Verification items for the finished model (mm, model axes). Face numbers are marked on the shaded views. A direction names the side the tool comes from. Give positions to 0.01 mm unless a question says otherwise; leave off trailing zeros. Write each loop counter-clockwise with the first axis right and the second up, starting at its lowest first coordinate (ties: lowest second). Pieces come first, ordered by that corner, then holes. Notation, with made-up numbers: (57.5, 83.25) - (66.5, 83.25) arc R8 ccw to (66.5, 93.25) - close; hole circle Ø10 at (82.25, 86). An arc over 180 degrees is marked (long way). Answer as a JSON object with one key per item and string values. Group by question number.
Item 1: Go/stop test with flat-tipped pins: pin 1 (3 mm diameter, centred on x = -6.5, y = -8, fed in from +Z); pin 2 (1 mm diameter, centred on y = -6, z = 33.5, fed in from -X); pin 3 (12 mm diameter, centred on x = 6, y = 8.5, fed in from +Z). Record where each tip stops, or that it passes through.
Item 2: Sectioned sample at D-D, the plane z = 50. Record the boundary of the cut face in (x, y), and give its area (3 significant figures).
Item 3: Sectioned sample at A-A, the plane x = 0. Record the boundary of the cut face in (y, z).
Item 4: Tool access check on the marked faces 1 and 2. Record the directions out of +Z, -Z, +X, -X, +Y, -Y that give a thin tool (end or side, any length) a straight path to the whole face; none if there is none.
Item 5: Scan lines: line 1 along Z through (x, y) = (11.5, 4.75); line 2 along Z through (x, y) = (-0.5, 3.5); line 3 along Y through (x, z) = (-8, 40.8). Record each from-to range of solid material in increasing order. Write a range as [from, to].
Item 6: Sectioned sample at B-B, the plane z = 14.5. Record the boundary of the cut face in (x, y), and give its area (3 significant figures).
Item 7: Sectioned sample at C-C, the plane y = 12.25. Record the boundary of the cut face in (x, z), and give its area (3 significant figures).
```python
from build123d import *

# Parameters (mm, degrees)
F0_R     = 14
F1_DEPTH = 42
F2_R     = 5
F3_DEPTH = 2.2
F4_R     = 2.25
F5_DEPTH = 17.25
F6_D     = 2.2
F6_DEPTH = 4
F6_TIP   = 0.6609466809


with BuildPart() as f1:
    # F0 (on Top) → F1 (new body)
    with BuildSketch(Plane.XY):
        Circle(F0_R)
    extrude(amount=F1_DEPTH)

    # F2 (on face) → F3 (join)
    with BuildSketch(Plane.XY.offset(42)):
        Circle(F2_R)
    extrude(amount=F3_DEPTH)

    # F4 (on face) → F5 (join)
    with BuildSketch(Plane.XY.offset(44.2)):
        Circle(F4_R)
    extrude(amount=F5_DEPTH)

    # F6
    with Locations(Plane.XY.offset(42)):
        with Locations((-8, 0), (8, 0)):
            Hole(F6_D / 2, depth=F6_DEPTH)
            with Locations((0, 0, -(F6_DEPTH + F6_TIP / 2))):  # 118° drill point
                Cone(0, F6_D / 2, F6_TIP, mode=Mode.SUBTRACT)


solid = f1.part
```
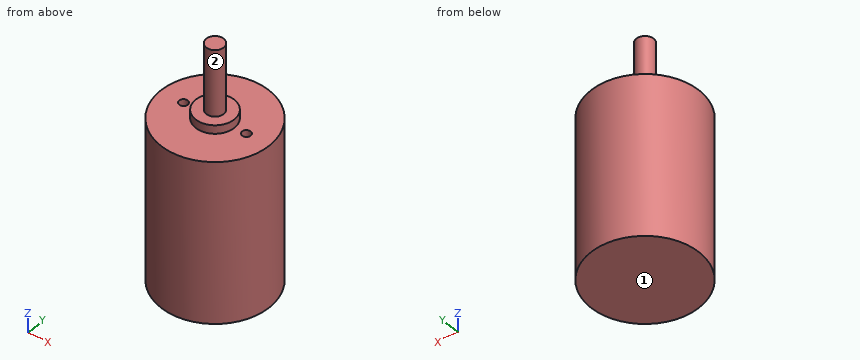
Geometry check:
{
 "1": {"pin 1": "z = 42", "pin 2": "x = -12.87", "pin 3": "z = 44.2"},
 "2": {"outline": "circle Ø4.5 at (0, 0)", "area": "15.9 mm^2"},
 "3": {"outline": "(-14, 0) - (14, 0) - (14, 42) - (5, 42) - (5, 44.2) - (2.25, 44.2) - (2.25, 61.45) - (-2.25, 61.45) - (-2.25, 44.2) - (-5, 44.2) - (-5, 42) - (-14, 42) - close"},
 "4": {"face 1": "-Z, +X, -X, +Y, -Y", "face 2": "+Z"},
 "5": {"line 1": "[0, 42]", "line 2": "[0, 44.2]", "line 3": "[-11.49, -1.1], [1.1, 11.49]"},
 "6": {"outline": "circle Ø28 at (0, 0)", "area": "616 mm^2"},
 "7": {"outline": "(-6.78, 0) - (6.78, 0) - (6.78, 42) - (-6.78, 42) - close", "area": "569 mm^2"}
}
